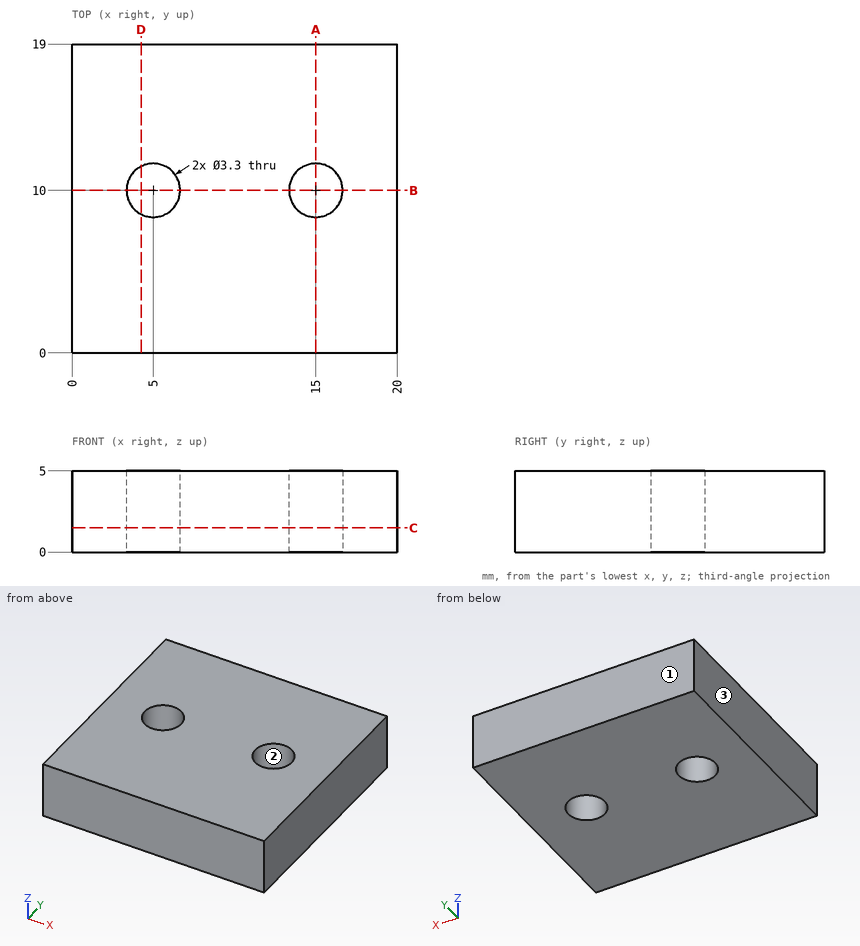
Input: dimensioned drawing with shaded views. Units: mm. Origin: part minimum x, y, z. Give positions to 0.01 mm unless a question says otherwise; leave off trailing zeros. Loops run counter-clockwise (first coordinate to the right, second up) from the corner with the lowest first, then second, coordinate; pieces in that order, holes last. Notation, with made-up numbers: (-31.75, -27) -> (-19.75, -27) arc R19 cw to (-19.75, -19) -> close; hole circle Ø3 at (82.5, -39.75). An arc over 180 degrees is marked (long way). Use a Markdown table: item, result.
Q1. Section query D-D, the plane x = 4.25. Return the cut outline in (y, z), plus the area to 3 significant figures.
Entries:
| item | result |
|---|---|
| outline | (0, 0) -> (8.53, 0) -> (8.53, 5) -> (0, 5) -> close; (11.47, 0) -> (19, 0) -> (19, 5) -> (11.47, 5) -> close |
| area | 80.3 mm² |
Q2. Section query A-A, the plane x = 15. Return the cut outline in (y, z).
Entries:
| item | result |
|---|---|
| outline | (0, 0) -> (8.35, 0) -> (8.35, 5) -> (0, 5) -> close; (11.65, 0) -> (19, 0) -> (19, 5) -> (11.65, 5) -> close |
Q3. Section query B-B, the plane y = 10. Return the cut outline in (x, z), plus the area to 3 significant figures.
Entries:
| item | result |
|---|---|
| outline | (0, 0) -> (3.35, 0) -> (3.35, 5) -> (0, 5) -> close; (6.65, 0) -> (13.35, 0) -> (13.35, 5) -> (6.65, 5) -> close; (16.65, 0) -> (20, 0) -> (20, 5) -> (16.65, 5) -> close |
| area | 67.0 mm² |
Q4. Section query C-C, the plane z = 1.5. Return the cut outline in (x, y), plus the area to 3 significant figures.
Entries:
| item | result |
|---|---|
| outline | (0, 0) -> (20, 0) -> (20, 19) -> (0, 19) -> close; hole circle Ø3.3 at (5, 10); hole circle Ø3.3 at (15, 10) |
| area | 363 mm² |
Q5. Ray query, probe 1 along Y at (x, z) = (15, 3.3); probe 2 along Y at (x, z) = (3.5, 4.5). Return the intervals inside material, ascending. Write a range as from..to.
Entries:
| item | result |
|---|---|
| probe 1 | y = 0..8.35, 11.65..19 |
| probe 2 | y = 0..9.31, 10.69..19 |
Q6. First-contact query: P1, Ø2, axis at x = 5, y = 10, coming from the -Z side. Flat tip, straight axial feed; report the tip coordinate or a pass-through.
Entries:
| item | result |
|---|---|
| P1 | passes through |
Q7. Pull-direction query (X, two-part tool) for the marked faces 1, 2 and 3; classes: pulls with the +X half, pulls with the -X half, needs draft (parallel to the pull), parting line crosses it, or undercut.
Entries:
| item | result |
|---|---|
| face 1 | needs draft |
| face 2 | undercut |
| face 3 | pulls with the -X half |
